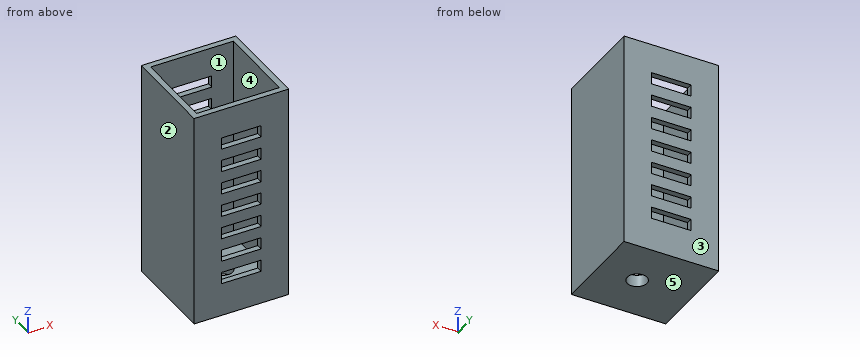
```python
from build123d import *

# Parameters (mm, degrees)
SKETCH007_W          = 21
SKETCH007_H          = 21
SKETCH007_R          = 2.5
PAD006_DEPTH         = 3
SKETCH008_W          = 24
SKETCH008_H          = 24
SKETCH008_W_2        = 21
SKETCH008_H_2        = 21
PAD007_DEPTH         = 55
SKETCH009_W          = 10
SKETCH009_H          = 3
POCKET001_DEPTH      = 20
POCKET001_DEPTH_BACK = 20
LINEARPATTERN_COUNT  = 7
LINEARPATTERN_PITCH  = 6


with BuildPart() as part:
    # Sketch007 → Pad006 (new body)
    with BuildSketch(Plane.XY):
        Rectangle(SKETCH007_W, SKETCH007_H)
        with Locations((2, 0)):
            Circle(SKETCH007_R, mode=Mode.SUBTRACT)
    extrude(amount=PAD006_DEPTH)

    # Sketch008 → Pad007 (join)
    with BuildSketch(Plane.XY):
        Rectangle(SKETCH008_W, SKETCH008_H)
        Rectangle(SKETCH008_W_2, SKETCH008_H_2, mode=Mode.SUBTRACT)
    extrude(amount=PAD007_DEPTH)

    # Sketch009 → Pocket001 (cut, two sides)
    with BuildSketch(Plane.XZ) as pocket001_sk:
        with Locations((0, 10)):
            Rectangle(SKETCH009_W, SKETCH009_H)
    pocket001 = extrude(amount=-POCKET001_DEPTH, mode=Mode.SUBTRACT) + extrude(pocket001_sk.sketch, amount=POCKET001_DEPTH_BACK, mode=Mode.SUBTRACT)

    # LinearPattern: Pocket001 ×7
    with Locations(*[(0, 0, i * LINEARPATTERN_PITCH) for i in range(1, LINEARPATTERN_COUNT)]):
        add(pocket001, mode=Mode.SUBTRACT)


with BuildPart() as part_1:
    # Body002 placement: moved
    add(part.part.moved(Location((0, 0, 20.5))))


solid = part_1.part
```
Build history of the part. All positions in model axes, mm. Face numbers are marked on the shaded views. A direction names the side the tool comes from. Round coordinates to 2 decimals unless told otherwise and drop trailing zeros. Order: outer loops, then holes, each group sorted by start corner. A loop starts at its lowest first (then second) coordinate and runs counter-clockwise, first axis right, second up. Notation, with made-up numbers: (-32, 66.5) - (3, 66.5) arc R14 ccw to (3, 89.5) - close; hole circle Ø4 at (79.25, 25.25). An arc over 180 degrees is marked (long way). Use a Markdown table: item, result.
1) Saw through at C-C on x = 2. Give the number of separate pieces and of enclosed holes in the cut face, and give its area (3 significant figures).
Recorded:
| item | result |
|---|---|
| separate pieces | 16 |
| enclosed holes | 0 |
| area | 150 mm² |
2) Saw through at A-A on y = 0. Write the cut outline in (x, z).
Recorded:
| item | result |
|---|---|
| outline | (-12, 20.5) - (-0.5, 20.5) - (-0.5, 23.5) - (-10.5, 23.5) - (-10.5, 75.5) - (-12, 75.5) - close; (4.5, 20.5) - (12, 20.5) - (12, 75.5) - (10.5, 75.5) - (10.5, 23.5) - (4.5, 23.5) - close |
3) Saw through at D-D on y = 8.75. Write the cut outline in (x, z), and give its area (3 significant figures).
Recorded:
| item | result |
|---|---|
| outline | (-12, 20.5) - (12, 20.5) - (12, 75.5) - (10.5, 75.5) - (10.5, 23.5) - (-10.5, 23.5) - (-10.5, 75.5) - (-12, 75.5) - close |
| area | 228 mm² |
4) Wall check: L1, parallel to Y at x = 10, z = 64; L2, parallel to Z at x = -3, y = -5.75. Give the ranges that are in metal, low to high.
Recorded:
| item | result |
|---|---|
| L1 | y = -12 to -10.5, 10.5 to 12 |
| L2 | z = 20.5 to 23.5 |
5) Tool access for the marked faces 4 and 5: list every direction of +Z, -Z, +X, -X, +Y, -Y with a clear straight run to the whole face (end or side of a thin tool).
Recorded:
| item | result |
|---|---|
| face 4 | +Z |
| face 5 | -Z, +X, -X, +Y, -Y |
6) Pull direction Y, two halves, no side cores. Call the marked faces 1, 2 and 3: pulls with the +Y half, pulls with the -Y half, needs draft (parallel to the pull), parting line crosses it, or undercut.
Recorded:
| item | result |
|---|---|
| face 1 | undercut |
| face 2 | needs draft |
| face 3 | pulls with the +Y half |
7) Flat gauge pin, fed straight in: pin 1 Ø5 at (x, y) = (-4, -7.5) entering from +Z. Where does the tip first touch, or does it go through?
Recorded:
| item | result |
|---|---|
| pin 1 | stops at z = 23.5 |
8) Saw through at B-B on z = 72.5. Write the cut outline in (x, y).
Recorded:
| item | result |
|---|---|
| outline | (-12, -12) - (12, -12) - (12, 12) - (-12, 12) - close; hole (-10.5, -10.5) - (10.5, -10.5) - (10.5, 10.5) - (-10.5, 10.5) - close |
